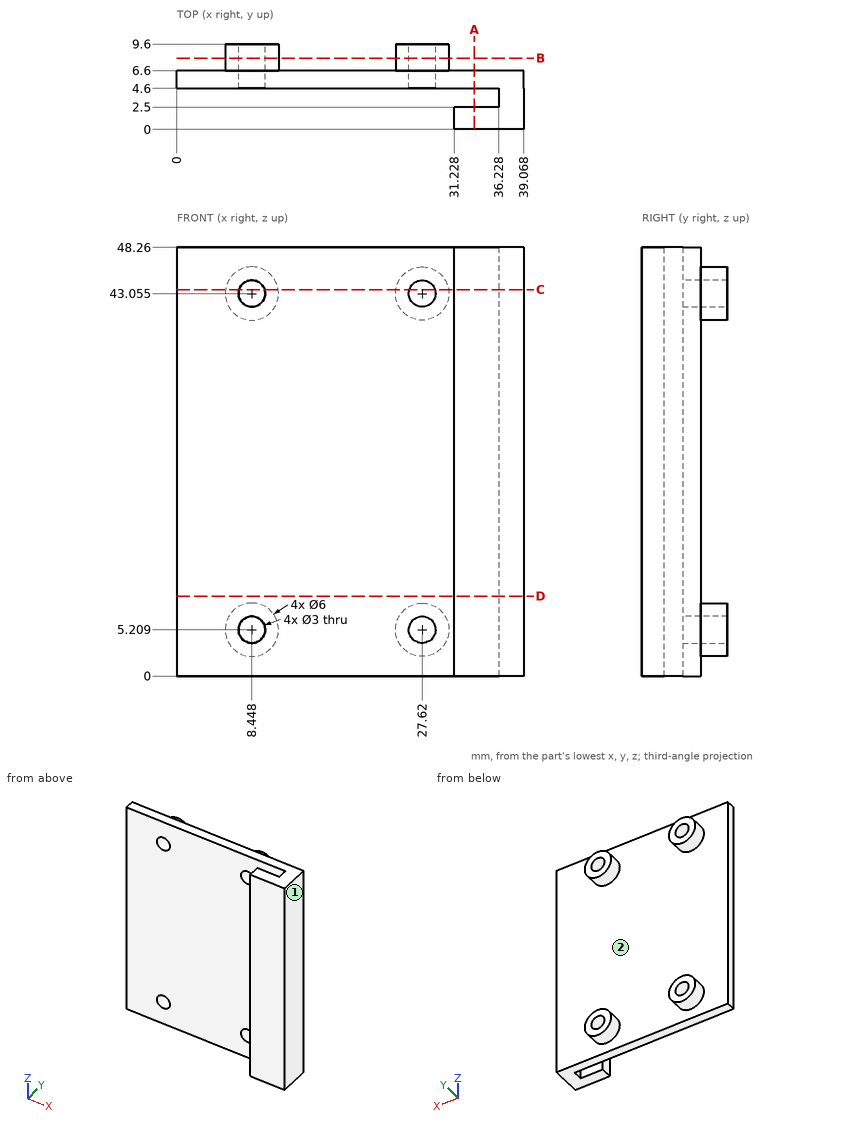
For this review, use the dimensioned drawing (mm, ordinates from the lowest corner) and the shaded views. A direction names the side the tool comes from. Coordinates: 2 decimals unless noted, no trailing zeros. Write each loop counter-clockwise with the first axis right and the second up, starting at its lowest first coordinate (ties: lowest second). Pieces come first, ordered by that corner, then holes. Notation, with made-up numbers: (28.25, -11.5) -> (66.25, -11.5) arc R30 cw to (66.25, 17.5) -> close; hole circle Ø9 at (-8.75, 47). An arc over 180 degrees is marked (long way). Write each question's results on one line, items separated by ' | '. Start each with the question number.
(1) Clearance check with flat-ended pins moving along their axes: P1, Ø1, axis at x = 25.5, y = 4.5, coming from the +Z side; P2, Ø0.6, axis at y = 3.5, z = 33, coming from the -X side; P3, Ø6, axis at x = 25, z = 16.5, coming from the -Y side; P4, Ø5.5, axis at x = 33.5, z = 15.5, coming from the +Y side. State where each tip first meets the part, or that it passes through.
(2) Take a section at A-A on x = 33.5. Write out the cut boundary in (y, z), and give its area (3 significant figures).
(3) For line 1 along Y through (x, z) = (13, 25.5); line 2 along X through (y, z) = (4, 22); line 3 along Y through (x, z) = (36, 26.5), list the stretches that pass through material, from the lowest coordinate up. Write a range as from..to.
(4) Take a section at D-D on z = 9. Write out the cut boundary in (x, y).
(5) Take a section at B-B on y = 8. Write out the cut boundary in (x, z) (1 decimal).
(6) Tool access review of the marked faces 1 and 2: name each direction out of +Z, -Z, +X, -X, +Y, -Y from which nothing blocks a thin tool from reaching the whole face with its end or side.
(7) Take a section at C-C on z = 43.5. Write out the cut boundary in (x, y) (1 decimal).
Results found:
1) P1: stops at z = 48.26 | P2: stops at x = 36.23 | P3: stops at y = 4.6 | P4: stops at y = 6.6
2) outline: (0, 0) -> (2.5, 0) -> (2.5, 48.26) -> (0, 48.26) -> close; (4.6, 0) -> (6.6, 0) -> (6.6, 48.26) -> (4.6, 48.26) -> close | area: 217 mm2
3) line 1: y = 4.6..6.6 | line 2: x = 36.23..39.07 | line 3: y = 0..2.5, 4.6..6.6
4) outline: (0, 4.6) -> (36.23, 4.6) -> (36.23, 2.5) -> (31.23, 2.5) -> (31.23, 0) -> (39.07, 0) -> (39.07, 6.6) -> (0, 6.6) -> close
5) outline: circle Ø6 at (8.4, 5.2); circle Ø6 at (8.4, 43.1); circle Ø6 at (27.6, 5.2); circle Ø6 at (27.6, 43.1); hole circle Ø3 at (8.4, 5.2); hole circle Ø3 at (8.4, 43.1); hole circle Ø3 at (27.6, 5.2); hole circle Ø3 at (27.6, 43.1)
6) face 1: +Z, -Z, +X, +Y, -Y | face 2: +Y
7) outline: (0, 4.6) -> (7, 4.6) -> (7, 9.6) -> (5.5, 9.6) -> (5.5, 6.6) -> (0, 6.6) -> close; (9.9, 4.6) -> (26.2, 4.6) -> (26.2, 9.6) -> (24.7, 9.6) -> (24.7, 6.6) -> (11.4, 6.6) -> (11.4, 9.6) -> (9.9, 9.6) -> close; (29.1, 4.6) -> (36.2, 4.6) -> (36.2, 2.5) -> (31.2, 2.5) -> (31.2, 0) -> (39.1, 0) -> (39.1, 6.6) -> (30.6, 6.6) -> (30.6, 9.6) -> (29.1, 9.6) -> close
